```python
from build123d import *

# Parameters (mm, degrees)
RESSALTO_EXTRUS_O1_DEPTH = 20
ESBO_O2_R                = 1.5
CORTE_EXTRUS_O1_DEPTH    = 61.731016524
CORTE_EXTRUS_O2_DEPTH    = 61.731016524


with BuildPart() as part:
    # Esboço1 → Ressalto-extrusão1 (new body)
    with BuildSketch(Plane.XY):
        with BuildLine():
            Line((-54.948124335, 11.894856768), (-45.448124335, 11.894856768))
            ThreePointArc((-45.448124335, 11.894856768), (-32.948124335, -0.605143232), (-20.448124335, 11.894856768))
            Line((-20.448124335, 11.894856768), (-10.948124335, 11.894856768))
            Line((-10.948124335, 11.894856768), (-10.948124335, 7.894856768))
            Line((-10.948124335, 7.894856768), (-17.043408054, 7.894856768))
            ThreePointArc((-17.043408054, 7.894856768), (-32.948124335, -4.505143232), (-48.852840617, 7.894856768))
            Line((-48.852840617, 7.894856768), (-54.948124335, 7.894856768))
            Line((-54.948124335, 7.894856768), (-54.948124335, 11.894856768))
        make_face()
    extrude(amount=RESSALTO_EXTRUS_O1_DEPTH)

    # Esboço2 → Corte-extrusão1 (cut, through all)
    with BuildSketch(Plane(origin=(0, 11.894856768, 0), x_dir=(1, 0, 0), z_dir=(0, 1, 0))):
        with Locations(Location((-51.698124335, -5, 0), (0, 0, 270))):
            Circle(ESBO_O2_R)
        with Locations(Location((-51.698124335, -15, 0), (0, 0, 270))):
            Circle(ESBO_O2_R)
        with Locations(Location((-14.198124335, -5, 0), (0, 0, 270))):
            Circle(ESBO_O2_R)
        with Locations(Location((-14.198124335, -15, 0), (0, 0, 270))):
            Circle(ESBO_O2_R)
    extrude(amount=-CORTE_EXTRUS_O1_DEPTH, mode=Mode.SUBTRACT)

    # Esboço3 → Corte-extrusão2 (cut, through all)
    with BuildSketch(Plane(origin=(0, 11.894856768, 0), x_dir=(1, 0, 0), z_dir=(0, 1, 0))):
        Polygon((-10.948124335, -21.140031795), (-8.775432295, -20.480907324), (-9.177542531, -19.85151739), (-10.948124335, -19), (-12.948124335, -20), (-13.238837314, -21.140031795), align=None)
        Polygon((-54.948124335, -19), (-52.948124335, -20), (-52.948124335, -22.628376124), (-56.762312397, -22.628376124), (-56.762312397, -19), align=None)
    extrude(amount=-CORTE_EXTRUS_O2_DEPTH, mode=Mode.SUBTRACT)


solid = part.part
```
Input: part model. Units: mm. Frame: model coordinates. A direction names the side the tool comes from. Round coordinates to 2 decimals unless told otherwise and drop trailing zeros. Order: outer loops, then holes, each group sorted by start corner. A loop starts at its lowest first (then second) coordinate and runs counter-clockwise, first axis right, second up. Notation, with made-up numbers: (75.25, 52) - (93.25, 52) arc R13 ccw to (93.25, 70) - close; hole circle Ø8 at (30.25, 28). An arc over 180 degrees is marked (long way). Answer in a Markdown table with one row per item.
Item 1: Section query A-A (z = 5). Return the cut outline in (x, y).
Model answer:
| item | result |
|---|---|
| outline | (-54.95, 7.89) - (-53.2, 7.89) - (-53.2, 11.89) - (-54.95, 11.89) - close; (-50.2, 7.89) - (-48.85, 7.89) arc R16.4 ccw to (-17.04, 7.89) - (-15.7, 7.89) - (-15.7, 11.89) - (-20.45, 11.89) arc R12.5 cw to (-45.45, 11.89) - (-50.2, 11.89) - close; (-12.7, 7.89) - (-10.95, 7.89) - (-10.95, 11.89) - (-12.7, 11.89) - close |
Item 2: Mould query, pull axis X, two halves, no side actions, for faces 4 (the flat face through (-34, -1, 0)), 5 (the cylindrical face through (-13.184, 9.923, 13.894)), 6 (the cylindrical face through (-32.6, -4.5, 9.9)). Classes: released by +X, released by -X, zero draft, split by the parting line, or undercut.
Model answer:
| item | result |
|---|---|
| face 4 | zero draft |
| face 5 | undercut |
| face 6 | split by the parting line |
Item 3: Line query: line 1 (X direction, y = 10.6, z = 5); line 2 (X direction, y = 9.65, z = 5); line 3 (X direction, y = 2, z = 2.5). Output: solid intervals per line, ascending.
Model answer:
| item | result |
|---|---|
| line 1 | x = -54.95 to -53.2, -50.2 to -45.38, -20.52 to -15.7, -12.7 to -10.95 |
| line 2 | x = -54.95 to -53.2, -50.2 to -45.24, -20.65 to -15.7, -12.7 to -10.95 |
| line 3 | x = -46.03 to -40.59, -25.31 to -19.87 |
Item 4: Section query D-D (z = 12.25). Return the cut outline in (x, y).
Model answer:
| item | result |
|---|---|
| outline | (-54.95, 7.89) - (-48.85, 7.89) arc R16.4 ccw to (-17.04, 7.89) - (-10.95, 7.89) - (-10.95, 11.89) - (-20.45, 11.89) arc R12.5 cw to (-45.45, 11.89) - (-54.95, 11.89) - close |
Item 5: Section query B-B (y = 10.5). Return the cut outline in (x, z), then the cut area to 3 significant figures.
Model answer:
| item | result |
|---|---|
| outline | (-54.95, 0) - (-45.37, 0) - (-45.37, 20) - (-52.95, 20) - (-54.95, 19) - close; (-20.53, 0) - (-10.95, 0) - (-10.95, 19) - (-12.95, 20) - (-20.53, 20) - close; hole circle Ø3 at (-51.7, 5); hole circle Ø3 at (-51.7, 15); hole circle Ø3 at (-14.2, 5); hole circle Ø3 at (-14.2, 15) |
| area | 353 mm² |
Item 6: Reachability of faces 1 (the cylindrical face through (-50.684, 9.923, 13.894)), 2 (the flat face through (-14, 7.895, 10)), 3 (the flat face through (-52, 7.895, 10)) from +Z, -Z, +X, -X, +Y, -Y: full face, straight path, thin tool, end or side. Return the list, or none.
Model answer:
| item | result |
|---|---|
| face 1 | +Y, -Y |
| face 2 | +Z, -Z, +X, -Y |
| face 3 | +Z, -Z, -X, -Y |
Item 7: Section query C-C (y = 7). Return the cut outline in (x, z), then the cut area to 3 significant figures.
Model answer:
| item | result |
|---|---|
| outline | (-48.6, 0) - (-44.45, 0) - (-44.45, 20) - (-48.6, 20) - close; (-21.45, 0) - (-17.3, 0) - (-17.3, 20) - (-21.45, 20) - close |
| area | 166 mm² |
Item 8: Pin query (flat end, axial travel): pin 1 (3 mm diameter, centred on x = -52, z = 7, fed in from -Y); pin 2 (5 mm diameter, centred on x = -50.5, z = 9, fed in from -Y); pin 3 (10 mm diameter, centred on x = -49, z = 11, fed in from -Y). Return the tip coordinate at first contact, or that it passes through.
Model answer:
| item | result |
|---|---|
| pin 1 | stops at y = 7.89 |
| pin 2 | stops at y = 5.38 |
| pin 3 | stops at y = -0.22 |
